Source: CAD feature listing. Evaluate the final solid. Frame: model axes, mm. Face numbers are marked on the shaded views. A direction names the side the tool comes from. Round coordinates to 2 decimals unless told otherwise and drop trailing zeros. Loops run counter-clockwise (first coordinate to the right, second up) from the corner with the lowest first, then second, coordinate; pieces in that order, holes last. Notation, with made-up numbers: (65, 9) - (119, 9) arc R20 cw to (119, 24) - close; hole circle Ø10 at (48, 45.5). An arc over 180 degrees is marked (long way). Write item = value, one per line. Start each with the question number.
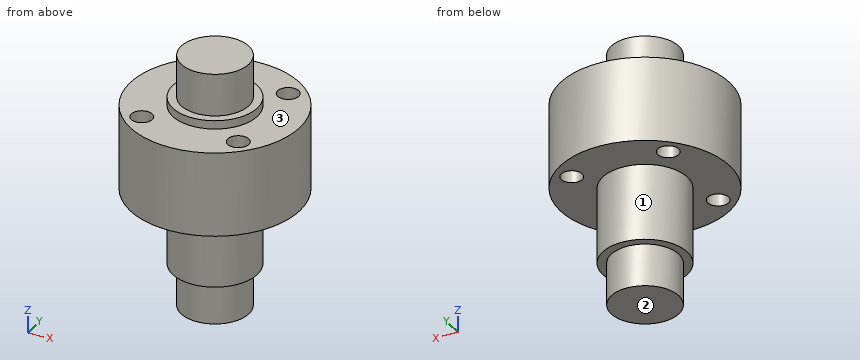
Autodesk Inventor part; units mm, degrees
ref_plane "YZ Plane" through (0, 0, 0) normal (1, 0, 0) x (0, 1, 0)
ref_plane "XZ Plane" through (0, 0, 0) normal (0, 1, 0) x (-1, 0, 0)
ref_plane "XY Plane" through (0, 0, 0) normal (0, 0, 1) x (1, 0, 0)
sketch "スケッチ1" plane through (0, 0, 0) normal (0, 0, 1) x (1, 0, 0)
  circle A0 centre (0, 0) radius 10
  dimension "d0" = 20
extrude "押し出し1" add sketch "スケッチ1" along normal blind 10
sketch "スケッチ2" plane through (0, 0, 10) normal (0, 0, 1) x (1, 0, 0)
  circle A0 centre (0, 0) radius 5
  dimension "d3" = 10
extrude "押し出し2" add sketch "スケッチ2" along normal blind 1
sketch "スケッチ3" plane through (0, 0, 11) normal (0, 0, 1) x (1, 0, 0)
  circle A0 centre (0, 0) radius 4
  dimension "d6" = 8
extrude "押し出し3" add sketch "スケッチ3" along normal blind 5
sketch "スケッチ4" plane through (0, 0, 0) normal (0, 0, -1) x (-1, 0, 0)
  circle A0 centre (0, 0) radius 5
  dimension "d9" = 10
extrude "押し出し4" add sketch "スケッチ4" along normal blind 9
sketch "スケッチ5" plane through (0, 0, -9) normal (0, 0, -1) x (-1, 0, 0)
  circle A0 centre (0, 0) radius 4
  dimension "d12" = 8
extrude "押し出し5" add sketch "スケッチ5" along normal blind 5
sketch "スケッチ6" plane through (0, 0, 0) normal (0, 0, -1) x (-1, 0, 0)
  circle A0 centre (0, 0) radius 8 construction
  line L0 (-5.6569, -5.6569) -> (5.6569, -5.6569) construction
  line L1 (5.6569, -5.6569) -> (5.6569, 5.6569) construction
  line L2 (5.6569, 5.6569) -> (-5.6569, 5.6569) construction
  line L3 (-5.6569, 5.6569) -> (-5.6569, -5.6569) construction
  line L4 (-5.6569, -5.6569) -> (5.6569, 5.6569) construction
  line L5 (5.6569, -5.6569) -> (-5.6569, 5.6569) construction
  dimension "d15" = 16
hole "穴1" at (-5.6569, 5.6569, 0) at (5.6569, 5.6569, 0) at (5.6569, -5.6569, 0) at (-5.6569, -5.6569, 0) direction (0, 0, 1) diameter 2.5 end through all
properties part number "AR20.0_wheel-shaft"
(1) Cut plane C-C (z = 7.75). Output: boundary loops of the cut face in (x, y), and give its area (3 significant figures).
(2) Cut plane D-D (y = 8.25). Output: boundary loops of the cut face in (x, z), and give its area (3 significant figures).
(3) Pin query (flat end, axial travel): P1, Ø6, axis at x = -7, z = -2.5, coming from the -Y side; P2, Ø1.5, axis at x = -3, y = -6, coming from the +Z side; P3, Ø1, axis at y = -7, z = 10, coming from the +X side. Return the tip coordinate at first contact, or that it passes through.
(4) Access query for the marked faces 1, 2 and 3. Directions: +Z, -Z, +X, -X, +Y, -Y. A direction counts if a zero-diameter tool reaches every point of the face in a straight line with its end or side. Return the directions, or none.
(5) Cut plane A-A (y = 0). Output: boundary loops of the cut face in (x, z).
(6) Material intervals for line 1 along Y through (x, z) = (6, 8.75); line 2 along Z through (x, y) = (2.75, 6.5); line 3 along X through (y, z) = (0.25, 9.25), sorted ascending. Write a range as from..to.
Solution:
q1.outline = circle Ø20 at (0, 0); hole circle Ø2.5 at (-5.66, -5.66); hole circle Ø2.5 at (-5.66, 5.66); hole circle Ø2.5 at (5.66, -5.66); hole circle Ø2.5 at (5.66, 5.66)
q1.area = 295 mm^2
q2.outline = (-5.65, 0) - (5.65, 0) - (5.65, 10) - (-5.65, 10) - close
q2.area = 113 mm^2
q3.P1 = -8.45
q3.P2 = 10
q3.P3 = 7.6
q4.face_1 = -Z
q4.face_2 = -Z, +X, -X, +Y, -Y
q4.face_3 = +Z
q5.outline = (-10, 0) - (-5, 0) - (-5, -9) - (-4, -9) - (-4, -14) - (4, -14) - (4, -9) - (5, -9) - (5, 0) - (10, 0) - (10, 10) - (5, 10) - (5, 11) - (4, 11) - (4, 16) - (-4, 16) - (-4, 11) - (-5, 11) - (-5, 10) - (-10, 10) - close
q6.line_1 = -8..-6.86, -4.45..4.45, 6.86..8
q6.line_2 = 0..10
q6.line_3 = -10..10
